The model under review builds one solid part; all positions refer to its coordinate system, in mm. A direction names the side the tool comes from. Coordinates: 2 decimals unless noted, no trailing zeros. Order: outer loops, then holes, each group sorted by start corner. A loop starts at its lowest first (then second) coordinate and runs counter-clockwise, first axis right, second up.
```python
from build123d import *

# Parameters (mm, degrees)
SKETCH1_R           = 12.7
SKETCH1_R_2         = 23.749
BOSS_EXTRUDE2_DEPTH = 2.54


with BuildPart() as part:
    # Sketch1 → Boss-Extrude2 (new body)
    with BuildSketch(Plane.YZ):
        with BuildLine():
            Line((0, 0), (0, 127))
            ThreePointArc((0, 127), (47.498, 174.498), (94.996, 127))
            Line((94.996, 127), (94.996, 0))
            ThreePointArc((94.996, 0), (47.498, -47.498), (0, 0))
        make_face()
        with Locations(Location((47.498, 0, 0), (0, 0, 270))):
            Circle(SKETCH1_R, mode=Mode.SUBTRACT)
        with Locations(Location((47.498, 127, 0), (0, 0, 270))):
            Circle(SKETCH1_R_2, mode=Mode.SUBTRACT)
        with BuildLine():
            Line((36.449, 90.551), (58.547, 90.551))
            ThreePointArc((58.547, 90.551), (67.527256121, 86.831256121), (71.247, 77.851))
            Line((71.247, 77.851), (71.247, 38.1))
            ThreePointArc((71.247, 38.1), (67.527256121, 29.119743879), (58.547, 25.4))
            Line((58.547, 25.4), (36.449, 25.4))
            ThreePointArc((36.449, 25.4), (27.468743879, 29.119743879), (23.749, 38.1))
            Line((23.749, 38.1), (23.749, 77.851))
            ThreePointArc((23.749, 77.851), (27.468743879, 86.831256121), (36.449, 90.551))
        make_face(mode=Mode.SUBTRACT)
    extrude(amount=BOSS_EXTRUDE2_DEPTH)


solid = part.part
```
(1) We need section C-C, the plane x = 0.4. Write out the cut boundary in (y, z), and give its area (3 significant figures).
A:
outline: (0, 0) arc R47.5 ccw to (95, 0) - (95, 127) arc R47.5 ccw to (0, 127) - close; hole (23.75, 38.1) arc R12.7 ccw to (36.45, 25.4) - (58.55, 25.4) arc R12.7 ccw to (71.25, 38.1) - (71.25, 77.85) arc R12.7 ccw to (58.55, 90.55) - (36.45, 90.55) arc R12.7 ccw to (23.75, 77.85) - close; hole circle Ø47.5 at (47.5, 127); hole circle Ø25.4 at (47.5, 0)
area: 13,900 mm2
(2) We need section A-A, the plane y = 53.5. Write out the cut boundary in (x, z).
A:
outline: (0, -47.12) - (2.54, -47.12) - (2.54, -11.19) - (0, -11.19) - close; (0, 11.19) - (2.54, 11.19) - (2.54, 25.4) - (0, 25.4) - close; (0, 90.55) - (2.54, 90.55) - (2.54, 104.02) - (0, 104.02) - close; (0, 149.98) - (2.54, 149.98) - (2.54, 174.12) - (0, 174.12) - close
(3) We need section B-B, the plane z = 134.5. Write out the cut boundary in (x, y).
A:
outline: (0, 0.6) - (2.54, 0.6) - (2.54, 24.96) - (0, 24.96) - close; (0, 70.03) - (2.54, 70.03) - (2.54, 94.4) - (0, 94.4) - close
(4) Machinability: for faces 4 (the face through (1.252, 48.542, -47.487)), 5 (the face through (1.25, 27.37, 86.73)), which of the approach directions +Z, -Z, +X, -X, +Y, -Y give a long, thin tool a straight path to every point of the face, cutting with its end or side? Answer none if there is none.
A:
face 4: -Z, +X, -X
face 5: +X, -X
(5) Wall thickness on probe 1 along Z at (x, y) = (2.4, 47); probe 2 along Y at (x, z) = (2.45, 59); probe 3 along Y at (x, z) = (0.35, 37.5): over which ranges is each line inside the solid? List them lowest first.
A:
probe 1: z = -47.5 to -12.69, 12.69 to 25.4, 90.55 to 103.26, 150.74 to 174.5
probe 2: y = 0 to 23.75, 71.25 to 95
probe 3: y = 0 to 23.76, 71.23 to 95
(6) For pin 1 Ø1.3 at (x, y) = (2, 43.5) entering from -Z; pin 2 Ø1 at (x, y) = (1, 72.5) entering from -Z; pin 3 Ø1.3 at (x, y) = (1, 47) entering from +Z; pin 4 Ø20.5 at (y, z) = (47.498, 0) entering from -X, all flat-tipped, find the tip position at first contact; note any pin that passes through.
A:
pin 1: stops at z = -47.38
pin 2: stops at z = -40.69
pin 3: stops at z = 174.5
pin 4: passes through
(7) We need section D-D, the plane y = 68. Write out the cut boundary in (x, z), and give its area (3 significant figures).
A:
outline: (0, -42.85) - (2.54, -42.85) - (2.54, 29.62) - (0, 29.62) - close; (0, 86.33) - (2.54, 86.33) - (2.54, 115.01) - (0, 115.01) - close; (0, 138.99) - (2.54, 138.99) - (2.54, 169.85) - (0, 169.85) - close
area: 335 mm2
(8) Draft analysis for pull direction Z (two halves, no side actions). For faces 1 (the face through (1.252, 46.454, 174.487)), 2 (the face through (2.54, 80, 65)), 3 (the face through (1.252, 54.632, 104.348)), state which applies: released by +Z, released by -Z, zero draft, split by the parting line, or undercut.
A:
face 1: released by +Z
face 2: zero draft
face 3: undercut
